Autodesk Fusion 360 part; units mm, degrees
sketch "Sketch1" plane through (0, 0, 0) normal (0, 0, 1) x (1, 0, 0)
  circle A0 centre (0, 0) radius 3.5
  line L0 (0, 0) -> (2, 0)
  line L1 (2, 0) -> (2, 2)
  line L2 (2, 2) -> (-2, 2)
  line L3 (-2, 2) -> (-2, -2)
  line L4 (-2, -2) -> (2, -2)
  line L5 (2, -2) -> (2, 0)
  dimension "d1" = 7
  dimension "d2" = 2
  dimension "d3" = 2
  dimension "d4" = 4
  dimension "d5" = 4
  dimension "d6" = 4
  dimension "d7" = 2
extrude "Extrude1" add sketch "Sketch1" along normal blind 1
equation "d3 = d2"
equation "d4 = d2 * 2"
equation "d5 = d2 * 2"
equation "d6 = d2 * 2"
equation "d7 = d2"
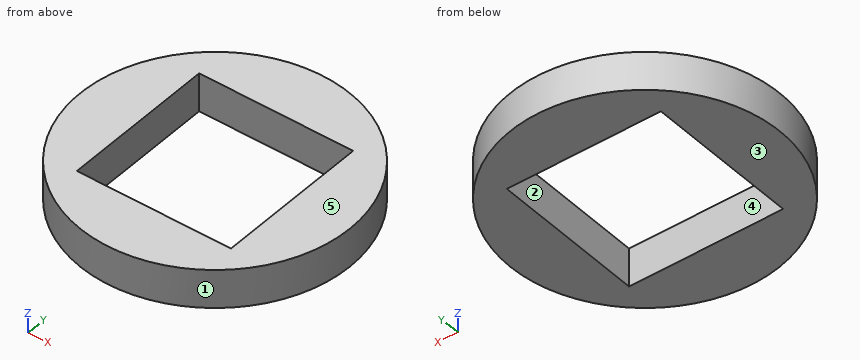
Part model, mm, in its own coordinate system. Face numbers are marked on the shaded views. A direction names the side the tool comes from. Coordinates: 2 decimals unless noted, no trailing zeros. Order: outer loops, then holes, each group sorted by start corner. A loop starts at its lowest first (then second) coordinate and runs counter-clockwise, first axis right, second up.
(1) Tool access for the marked faces 4 and 5: list every direction of +Z, -Z, +X, -X, +Y, -Y with a clear straight run to the whole face (end or side of a thin tool).
Check sheet entries:
face 4: +Z, -Z
face 5: +Z, +X, -X, +Y, -Y
(2) Slice it at C-C, the plane z = 0.35. Write the cut outline in (x, y), and give its area (3 significant figures).
Check sheet entries:
outline: circle Ø7 at (0, 0); hole (-2, -2) - (2, -2) - (2, 2) - (-2, 2) - close
area: 22.5 mm2
(3) Slice it at D-D, the plane x = 3. Write the cut outline in (y, z).
Check sheet entries:
outline: (-1.8, 0) - (1.8, 0) - (1.8, 1) - (-1.8, 1) - close
(4) Slice it at A-A, the plane y = 0. Write the cut outline in (x, z), and give its area (3 significant figures).
Check sheet entries:
outline: (-3.5, 0) - (-2, 0) - (-2, 1) - (-3.5, 1) - close; (2, 0) - (3.5, 0) - (3.5, 1) - (2, 1) - close
area: 3.00 mm2
(5) Probe L1, parallel to Y at x = 0, z = 0.65; L2, parallel to X at y = 1, z = 0.3; L3, parallel to X at y = 0.5, z = 0.3. List the from-to ranges inside material, lowest first.
Check sheet entries:
L1: y = -3.5 to -2, 2 to 3.5
L2: x = -3.35 to -2, 2 to 3.35
L3: x = -3.46 to -2, 2 to 3.46
(6) Pull direction Y, two halves, no side cores. Call the marked faces 1, 2 and 3: pulls with the +Y half, pulls with the -Y half, needs draft (parallel to the pull), parting line crosses it, or undercut.
Check sheet entries:
face 1: parting line crosses it
face 2: undercut
face 3: needs draft
